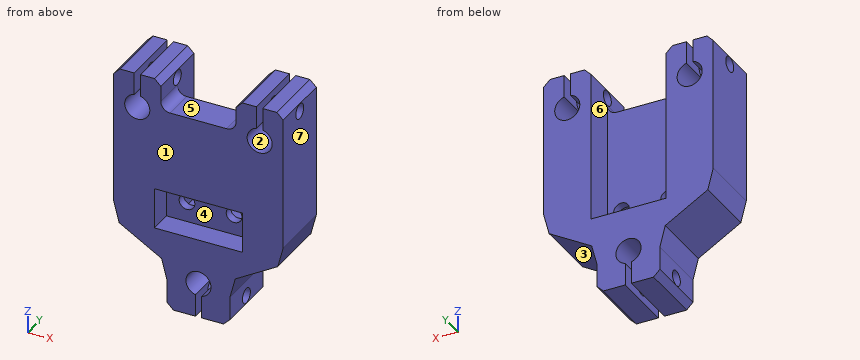
```python
from build123d import *

# Parameters (mm, degrees)
SKETCH1_W             = 24
SKETCH1_H             = 40
SKETCH1_R             = 2.5
BOSS_EXTRUDE1_DEPTH   = 10
SKETCH2_R             = 4
BOSS_EXTRUDE2_DEPTH   = 20
SKETCH4_W             = 2
SKETCH4_H             = 15
CUT_EXTRUDE1_DEPTH    = 20
SKETCH5_R             = 2.4
CUT_EXTRUDE2_DEPTH    = 56
CHAMFER2_SIZE         = 2
CHAMFER3_SIZE2        = 2
CHAMFER3_SIZE         = 5.63516655
CHAMFER3_EDGE_2_SIZE2 = 5.63516655
CHAMFER3_EDGE_2_SIZE  = 2
CHAMFER3_EDGE_3_SIZE2 = 2
CHAMFER3_EDGE_3_SIZE  = 5.63516655
CHAMFER3_EDGE_4_SIZE2 = 5.63516655
CHAMFER3_EDGE_4_SIZE  = 2
FILLET2_R             = 3
SKETCH6_W             = 28
SKETCH6_H             = 13
CUT_EXTRUDE3_DEPTH    = 7.3


with BuildPart() as part:
    # Sketch1 → Boss-Extrude1 (new body)
    with BuildSketch(Plane(origin=(0, 0, 0), x_dir=(1, 0, 0), z_dir=(0, 1, 0))):
        Rectangle(SKETCH1_W, SKETCH1_H)
        with Locations((7.5, 13)):
            Circle(SKETCH1_R, mode=Mode.SUBTRACT)
        with Locations((-7.5, 13)):
            Circle(SKETCH1_R, mode=Mode.SUBTRACT)
    extrude(amount=BOSS_EXTRUDE1_DEPTH)

    # Sketch2 → Boss-Extrude2 (add)
    with BuildSketch(Plane.XZ):
        Polygon((-12, -20), (-12, 30), (-27, 30), (-27, -20), (-10, -30), (-10, -45), (10, -45), (10, -30), (27, -20), (27, 30), (12, 30), (12, -20), align=None)
        with Locations((0, -34)):
            Circle(SKETCH2_R, mode=Mode.SUBTRACT)
        with Locations((-19.5, 19)):
            Circle(SKETCH2_R, mode=Mode.SUBTRACT)
        with Locations((19.5, 19)):
            Circle(SKETCH2_R, mode=Mode.SUBTRACT)
    extrude(amount=-BOSS_EXTRUDE2_DEPTH)

    # Sketch4 → Cut-Extrude1 (cut)
    with BuildSketch(Plane(origin=(0, 20, 0), x_dir=(1, 0, 0), z_dir=(0, 1, 0))):
        with Locations((19.5, -30)):
            Rectangle(SKETCH4_W, SKETCH4_H)
        with Locations((-19.5, -30)):
            Rectangle(SKETCH4_W, SKETCH4_H)
        with Locations((0, 45)):
            Rectangle(SKETCH4_W, SKETCH4_H)
    extrude(amount=-CUT_EXTRUDE1_DEPTH, mode=Mode.SUBTRACT)

    # Sketch5 → Cut-Extrude2 (cut)
    with BuildSketch(Plane(origin=(27, 0, 0), x_dir=(0, 0, -1), z_dir=(1, 0, 0))):
        with Locations((-25.5, 10)):
            Circle(SKETCH5_R)
        with Locations((40.5, 10)):
            Circle(SKETCH5_R)
    extrude(amount=-CUT_EXTRUDE2_DEPTH, mode=Mode.SUBTRACT)

    # Chamfer2
    chamfer2_edges = [part.edges().sort_by_distance(p)[0] for p in [
        (12, 10, 30),
        (27, 10, 30),
        (10, 10, -45),
        (-10, 10, -45),
        (-27, 10, 30),
        (-12, 10, 30),
    ]]
    chamfer(chamfer2_edges, length=CHAMFER2_SIZE)

    # Chamfer3
    chamfer3_edges = [part.edges().sort_by_distance(p)[0] for p in [
        (27, 10, -20),
    ]]
    chamfer(chamfer3_edges, length=CHAMFER3_SIZE, length2=CHAMFER3_SIZE2)

    # Chamfer3 edge 2
    chamfer3_edge_2_edges = [part.edges().sort_by_distance(p)[0] for p in [
        (10, 10, -30),
    ]]
    chamfer(chamfer3_edge_2_edges, length=CHAMFER3_EDGE_2_SIZE, length2=CHAMFER3_EDGE_2_SIZE2)

    # Chamfer3 edge 3
    chamfer3_edge_3_edges = [part.edges().sort_by_distance(p)[0] for p in [
        (-10, 10, -30),
    ]]
    chamfer(chamfer3_edge_3_edges, length=CHAMFER3_EDGE_3_SIZE, length2=CHAMFER3_EDGE_3_SIZE2)

    # Chamfer3 edge 4
    chamfer3_edge_4_edges = [part.edges().sort_by_distance(p)[0] for p in [
        (-27, 10, -20),
    ]]
    chamfer(chamfer3_edge_4_edges, length=CHAMFER3_EDGE_4_SIZE, length2=CHAMFER3_EDGE_4_SIZE2)

    # Fillet2
    fillet2_edges = [part.edges().sort_by_distance(p)[0] for p in [
        (12, 5, 20),
        (-12, 5, 20),
    ]]
    fillet(fillet2_edges, radius=FILLET2_R)

    # Sketch6 → Cut-Extrude3 (cut)
    with BuildSketch(Plane.XZ):
        with Locations((0, -13)):
            Rectangle(SKETCH6_W, SKETCH6_H)
    extrude(amount=-CUT_EXTRUDE3_DEPTH, mode=Mode.SUBTRACT)


solid = part.part
```
Could you check a few things on this model? Use its own coordinates, in mm. Face numbers are marked on the shaded views. A direction names the side the tool comes from. Coordinates: 2 decimals unless noted, no trailing zeros. Write each loop counter-clockwise with the first axis right and the second up, starting at its lowest first coordinate (ties: lowest second). Pieces come first, ordered by that corner, then holes. Notation, with made-up numbers: (72, 70) -> (130, 70) arc R21 cw to (130, 105) -> close; hole circle Ø3 at (10, -34). An arc over 180 degrees is marked (long way). Return JSON: item names as keys, results as strings.
(1) Which directions (+Z, -Z, +X, -X, +Y, -Y) give clear straight access to the entire face, cutting with the end or side of a thin tool? Please do the marked faces 4, 5, 6 and 7.
Numbers:
{"face 4": "-Y", "face 5": "+Z, +Y, -Y", "face 6": "+Z, +Y", "face 7": "+Z, -Z, +X, +Y, -Y"}
(2) Imagine slicing it at D-D, the plane z = -31.5. Please give me the cut outline in (x, y), then the cut area to 3 significant figures.
Numbers:
{"outline": "(-11.07, 0) -> (-3.12, 0) -> (-3.12, 20) -> (-11.07, 20) -> close; (3.12, 0) -> (11.07, 0) -> (11.07, 20) -> (3.12, 20) -> close", "area": "318 mm2"}
(3) We'd pull the mould along Z, two halves only. Please class the marked faces 1, 2 and 3: +Z half, -Z half, draft (parallel to the pull), parting line (faces both ways), or undercut.
Numbers:
{"face 1": "draft", "face 2": "undercut", "face 3": "-Z half"}
(4) Imagine slicing it at A-A, the plane z = -40.5. Please give me the cut outline in (x, y), then the cut area to 3 significant figures.
Numbers:
{"outline": "(-10, 0) -> (-1, 0) -> (-1, 7.6) -> (-10, 7.6) -> close; (-10, 12.4) -> (-1, 12.4) -> (-1, 20) -> (-10, 20) -> close; (1, 0) -> (10, 0) -> (10, 7.6) -> (1, 7.6) -> close; (1, 12.4) -> (10, 12.4) -> (10, 20) -> (1, 20) -> close", "area": "274 mm2"}
(5) I need wall thicknesses on L1, parallel to X at y = 9.35, z = -13; L2, parallel to Z at x = -7.5, y = 5; L3, parallel to X at y = 13.25, z = -9. Which ranges of each line are inside material? Lowest first, please.
Numbers:
{"L1": "x = -27 to -10, -5 to 5, 10 to 27", "L2": "z = -45 to -19.5, -6.5 to 20", "L3": "x = -27 to -12, 12 to 27"}
(6) Imagine slicing it at B-B, the plane z = 19. Please give me the cut outline in (x, y), then the cut area to 3 significant figures.
Numbers:
{"outline": "(-27, 0) -> (-23.5, 0) -> (-23.5, 20) -> (-27, 20) -> close; (-15.5, 0) -> (15.5, 0) -> (15.5, 20) -> (12, 20) -> (12, 10) -> (-12, 10) -> (-12, 20) -> (-15.5, 20) -> close; (23.5, 0) -> (27, 0) -> (27, 20) -> (23.5, 20) -> close", "area": "520 mm2"}
(7) I'm going to push flat-ended pins straight in: pin 1 (3.5 mm diameter, centred on x = 1, y = 3, fed in from +Z); pin 2 (8 mm diameter, centred on x = -7.5, z = -13, fed in from +Y); pin 3 (8 mm diameter, centred on y = 14, z = -37, fed in from -X); pin 4 (10.5 mm diameter, centred on x = 0.5, z = -11.5, fed in from -Y). Where does each tip first touch, or does it pass through?
Numbers:
{"pin 1": "stops at z = 20", "pin 2": "stops at y = 10", "pin 3": "stops at x = -10.68", "pin 4": "stops at y = 0"}
(8) Imagine slicing it at C-C, the plane x = 0. Please give me the cut outline in (y, z), then the cut area to 3 significant figures.
Numbers:
{"outline": "(0, -30) -> (20, -30) -> (20, -20) -> (10, -20) -> (10, 20) -> (0, 20) -> (0, -6.5) -> (7.3, -6.5) -> (7.3, -19.5) -> (0, -19.5) -> close", "area": "505 mm2"}
